Can you work these out from the drawing? Everything is in mm from the part's minimum corner. A direction names the side the tool comes from. Round coordinates to 2 decimals unless told otherwise and drop trailing zeros. Write each loop counter-clockwise with the first axis right and the second up, starting at its lowest first coordinate (ties: lowest second). Pieces come first, ordered by that corner, then holes. Notation, with made-up numbers: (-36, -28) -> (-19, -28) arc R8 ccw to (-19, -21) -> close; hole circle Ø5 at (44, 72.5). An arc over 180 degrees is marked (long way). Put each result on its own line as item: value. Start each with the question number.
1. I need wall thicknesses on probe 1 along Y at (x, z) = (4.5, 11.25); probe 2 along Z at (x, y) = (7.5, 4.5) (1 decimal); probe 3 along X at (y, z) = (3.75, 12.75) (1 decimal). Which ranges of each line are inside material? Lowest first, please. Write a range as from..to.
2. For pin 1 (6.5 mm diameter, centred on x = 6.02, y = 11.2, fed in from +Z); pin 2 (1.5 mm diameter, centred on y = 9.5, z = 3.5, fed in from -X); pin 3 (3 mm diameter, centred on y = 10.5, z = 3, fed in from +X), each with a flat end and sliding along its axis, tell me the tip position at first contact or that it passes through.
3. Suppose I cut it at D-D (y = 11.2). Please give me the cut outline in (x, z) (1 decimal).
4. We'd pull the mould along Y, two halves only. Please class the marked faces 1, 2, 3 and 4: +Y half, -Y half, draft (parallel to the pull), parting line (faces both ways), or undercut.
5. Suppose I cut it at A-A (y = 1.25). Please give me the cut outline in (x, z) (1 decimal).
6. Which directions (+Z, -Z, +X, -X, +Y, -Y) give clear straight access to the entire face, cutting with the end or side of a thin tool? Please do the marked faces 5 and 6.
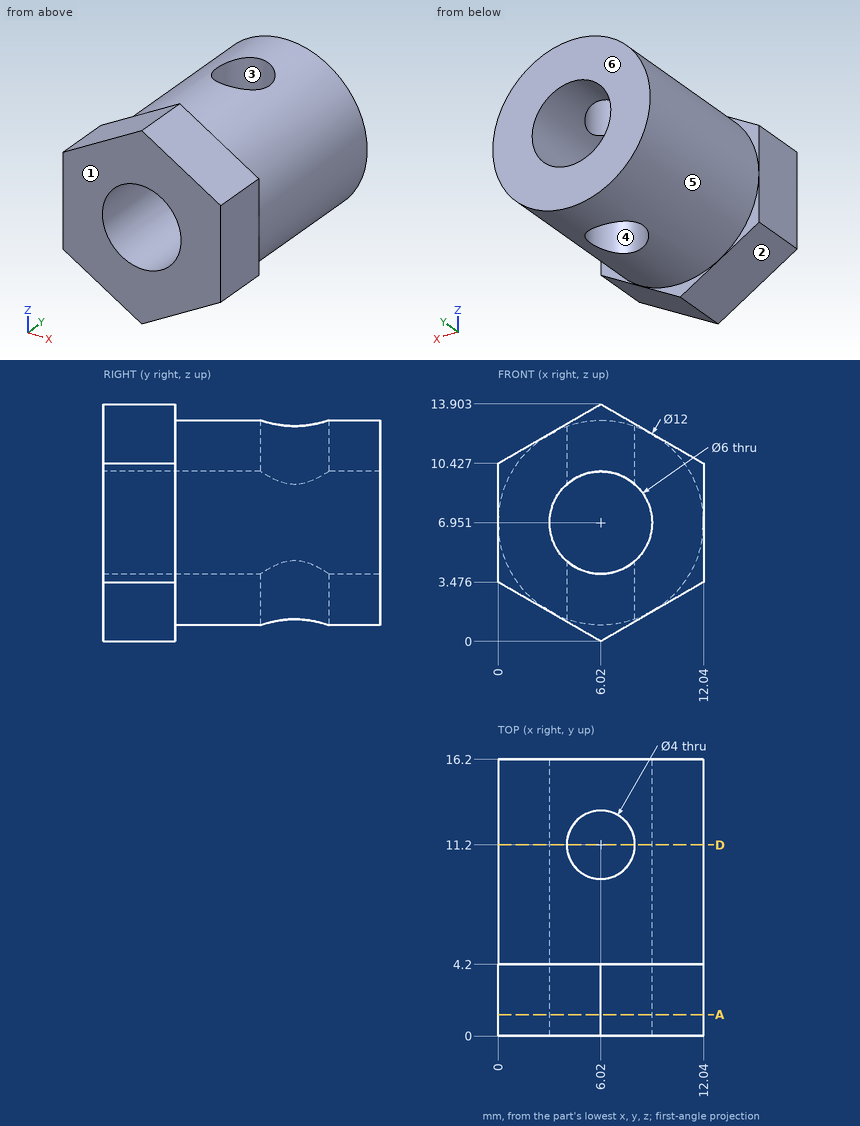
Verdict:
1. probe 1: y = 0..9.9, 12.5..16.2
1. probe 2: z = 1.1..4.3, 9.6..12.8
1. probe 3: x = 4..8
2. pin 1: stops at z = 12.95
2. pin 2: stops at x = 0.66
2. pin 3: stops at x = 11.5
3. outline: (4, 1.3) -> (4, 4.7) arc R3 cw to (4, 9.2) -> (4, 12.6) arc R6 ccw to start; (8, 1.3) arc R6 ccw to (8, 12.6) -> (8, 9.2) arc R3 cw to (8, 4.7) -> close
4. face 1: -Y half
4. face 2: draft
4. face 3: undercut
4. face 4: undercut
5. outline: (0, 3.5) -> (6, 0) -> (12, 3.5) -> (12, 10.4) -> (6, 13.9) -> (0, 10.4) -> close; hole circle Ø6 at (6, 7)
6. face 5: +Y
6. face 6: +Z, -Z, +X, -X, +Y
